Check sheet for the drawn part. Datum: minimum x, y, z corner. Units: mm. Coordinates: 2 decimals unless noted, no trailing zeros. Order: outer loops, then holes, each group sorted by start corner. A loop starts at its lowest first (then second) coordinate and runs counter-clockwise, first axis right, second up.
Q1. Cross-section at B-B, the plane z = 70. Record the boundary of the cut face in (x, y), and give its area (3 significant figures).
Q2. Thickness scan on line 1 (X direction, y = 5.5, z = 70); line 2 (X direction, y = 1.5, z = 70); line 3 (Z direction, x = 63, y = 1). Record the ranges inside material, lowest first.
Q3. Cross-section at C-C, the plane y = 5. Record the boundary of the cut face in (x, z) (1 decimal), and give its area (3 significant figures).
Q4. Cross-section at D-D, the plane x = 43. Record the boundary of the cut face in (y, z).
Q5. Depth check by flat-ended pin: P1, Ø10, axis at x = 84.5, z = 45, coming from the +Y side; P2, Ø2, axis at x = 97.5, y = 6, coming from the +Z side; P3, Ø3, axis at y = 1, z = 36, coming from the +X side. Enter the tip coordinate at first touch or a pass-through.
Q6. Cross-section at A-A, the plane x = 70. Record the boundary of the cut face in (y, z).
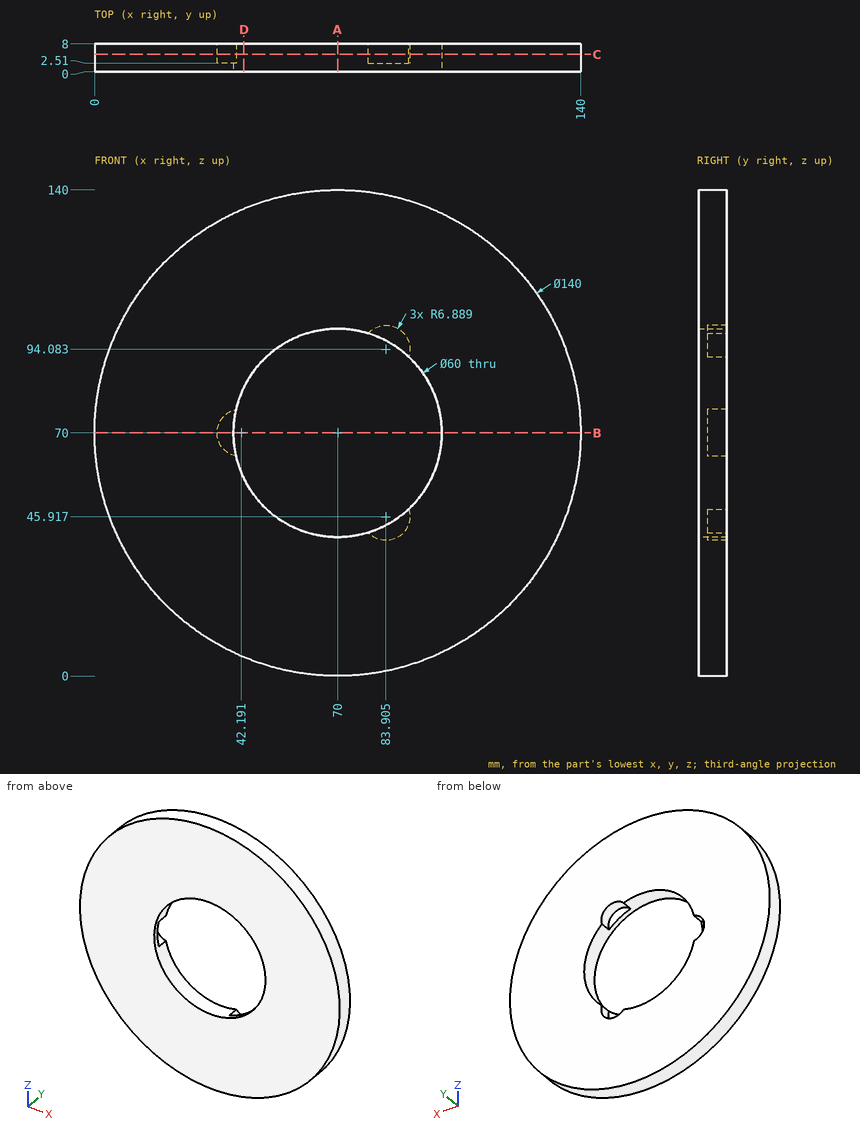
Check values:
1. outline: (0, 0) - (40, 0) - (40, 2.51) - (35.3, 2.51) - (35.3, 8) - (0, 8) - close; (100, 0) - (140, 0) - (140, 8) - (100, 8) - close
1. area: 614 mm2
2. line 1: x = 0 to 35.3, 100 to 140
2. line 2: x = 0 to 40, 100 to 140
2. line 3: z = 0.35 to 40.83, 99.17 to 139.65
3. outline: circle Ø140 at (70, 70); hole (40.8, 63.3) arc R30 ccw to (78.8, 41.3) arc R6.9 ccw to (90.5, 48.1) arc R30 ccw to (90.5, 91.9) arc R6.9 ccw to (78.8, 98.7) arc R30 ccw to (40.8, 76.7) arc R6.9 ccw to start
3. area: 12,400 mm2
4. outline: (0, 5.42) - (8, 5.42) - (8, 56.92) - (0, 56.92) - close; (0, 83.08) - (8, 83.08) - (8, 134.58) - (0, 134.58) - close
5. P1: stops at y = 2.51
5. P2: stops at z = 134.79
5. P3: stops at x = 132
6. outline: (0, 0) - (8, 0) - (8, 40) - (0, 40) - close; (0, 100) - (8, 100) - (8, 140) - (0, 140) - close
